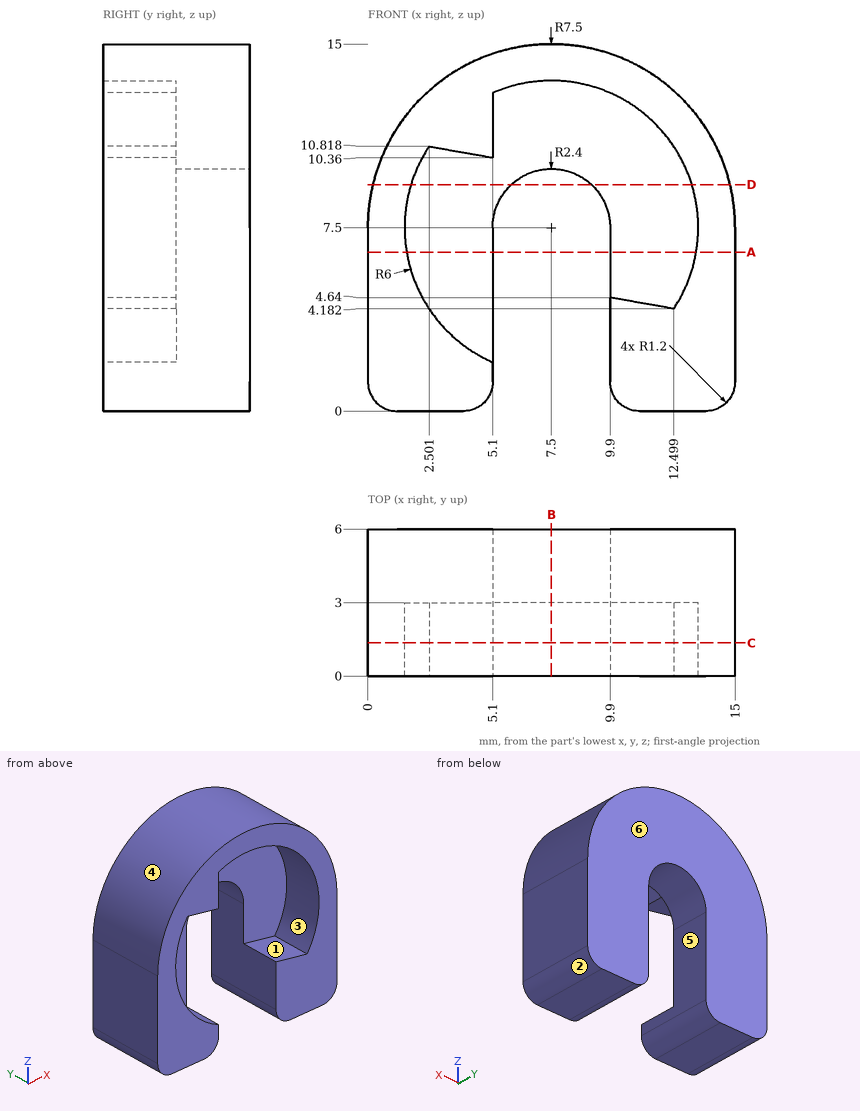
Source: three-view drawing plus pictorial views. Frame: mm from the lowest corner of the part. A direction names the side the tool comes from. Round coordinates to 2 decimals unless told otherwise and drop trailing zeros. Write each loop counter-clockwise with the first axis right and the second up, starting at its lowest first coordinate (ties: lowest second). Pieces come first, ordered by that corner, then holes. Notation, with made-up numbers: M 60,16 L 68,16 A17 cw 68,33 Z; hole C 22.5,22 d11. An arc over 180 degrees is marked long. One line per item, written item: value. Start each with the question number.
Item 1: Section query A-A (z = 6.5). Return the cut outline in (x, y), plus the area to 3 significant figures.
Item 2: Ray query, L1, parallel to X at y = 2.85, z = 2.5 (1 decimal); L2, parallel to X at y = 4.4, z = 5; L3, parallel to Y at x = 7.25, z = 13. Return the intervals inside material, ascending. Write a range as from..to.
Item 3: Section query B-B (x = 7.5). Return the cut outline in (y, z), plus the area to 3 significant figures.
Item 4: Pin query (flat end, axial travel): pin 1 (1 mm diameter, centred on x = 7, z = 2, fed in from -Y); pin 2 (3 mm diameter, centred on x = 8, y = 5, fed in from -Z) (1 decimal); pin 3 (0.8 mm diameter, centred on y = 1, z = 11.5, fed in from +X); pin 4 (2 mm diameter, centred on y = 4.5, z = 11, fed in from +X). Return the tip coordinate at first contact, or that it passes through.
Item 5: Section query C-C (y = 1.35). Return the cut outline in (x, z).
Item 6: Set-up query: the marked faces 5 and 6. Return all of +Z, -Z, +X, -X, +Y, -Y with unobstructed straight access to the full face (end or side cutting, diameter ignored); none if empty.
Item 7: Section query D-D (z = 9.25). Return the cut outline in (x, y).
Item 8: Mould query, pull axis X, two halves, no side actions, for the marked faces 1, 2, 3 and 4. Classes: pulls with the +X half, pulls with the -X half, needs draft (parallel to the pull), parting line crosses it, or undercut.
Result set:
1. outline: M 0,0 L 1.58,0 L 1.58,3 L 5.1,3 L 5.1,6 L 0,6 Z; M 9.9,3 L 13.42,3 L 13.42,0 L 15,0 L 15,6 L 9.9,6 Z
1. area: 40.1 mm²
2. L1: x = 0..4.2, 9.9..15
2. L2: x = 0..5.1, 9.9..15
2. L3: y = 3..6
3. outline: M 0,13.5 L 3,13.5 L 3,9.9 L 6,9.9 L 6,15 L 0,15 Z
3. area: 19.8 mm²
4. pin 1: passes through
4. pin 2: stops at z = 8.8
4. pin 3: stops at x = 14.08
4. pin 4: stops at x = 14.57
5. outline: M 0,1.2 A1.2 ccw 1.2,0 L 3.9,0 A1.2 ccw 5.1,1.2 L 5.1,2 A6 cw 2.5,10.82 L 5.1,10.36 L 5.1,13 A6 cw 12.5,4.18 L 9.9,4.64 L 9.9,1.2 A1.2 ccw 11.1,0 L 13.8,0 A1.2 ccw 15,1.2 L 15,7.5 A7.5 ccw 0,7.5 Z
6. face 5: -Z, +Y, -Y
6. face 6: +Z, -Z, +X, -X, +Y
7. outline: M 0.21,0 L 1.76,0 L 1.76,3 L 5.86,3 L 5.86,6 L 0.21,6 Z; M 9.14,3 L 13.24,3 L 13.24,0 L 14.79,0 L 14.79,6 L 9.14,6 Z
8. face 1: undercut
8. face 2: pulls with the +X half
8. face 3: undercut
8. face 4: parting line crosses it
